Could you check a few things on this model? Use its own coordinates, in mm. A direction names the side the tool comes from. Coordinates: 2 decimals unless noted, no trailing zeros. Loops run counter-clockwise (first coordinate to the right, second up) from the corner with the lowest first, then second, coordinate; pieces in that order, holes last. Notation, with made-up numbers: (86.25, 45.25) - (142.25, 45.25) arc R19 cw to (142.25, 57.25) - close; hole circle Ø9 at (24.25, 14). An arc over 180 degrees is marked (long way). Use CSV: the item, a comma, the result in double quotes.
from build123d import *

# Parameters (mm, degrees)
F1_DEPTH = 2.54
F3_DEPTH = 6.35
F4_W     = 80.137
F4_H     = 207.137
F5_DEPTH = 3.81


with BuildPart() as f1:
    # F0 (on Top) → F1 (new body)
    with BuildSketch(Plane.XY):
        with BuildLine():
            ThreePointArc((0, 1.27), (0.371974, 0.371974), (1.27, 0))
            Line((1.27, 0), (89.535, 0))
            ThreePointArc((89.535, 0), (90.433026, 0.371974), (90.805, 1.27))
            Line((90.805, 1.27), (90.805, 216.535))
            ThreePointArc((90.805, 216.535), (90.433026, 217.433026), (89.535, 217.805))
            Line((89.535, 217.805), (1.27, 217.805))
            ThreePointArc((1.27, 217.805), (0.371974, 217.433026), (0, 216.535))
            Line((0, 216.535), (0, 1.27))
        make_face()
    extrude(amount=F1_DEPTH)

    # F2 (on Top) → F3 (join)
    with BuildSketch(Plane.XY):
        with BuildLine():
            Line((2.794, 213.741), (2.794, 4.064))
            ThreePointArc((2.794, 4.064), (3.165974, 3.165974), (4.064, 2.794))
            Line((4.064, 2.794), (86.741, 2.794))
            ThreePointArc((86.741, 2.794), (87.639026, 3.165974), (88.011, 4.064))
            Line((88.011, 4.064), (88.011, 213.741))
            ThreePointArc((88.011, 213.741), (87.639026, 214.639026), (86.741, 215.011))
            Line((86.741, 215.011), (4.064, 215.011))
            ThreePointArc((4.064, 215.011), (3.165974, 214.639026), (2.794, 213.741))
        make_face()
    extrude(amount=F3_DEPTH)

    # F4 (on face) → F5 (cut)
    with BuildSketch(Plane.XY.offset(6.35)):
        with Locations((45.4025, 108.9025)):
            Rectangle(F4_W, F4_H)
    extrude(amount=-F5_DEPTH, mode=Mode.SUBTRACT)


solid = f1.part
(1) Suppose I cut it at B-B (y = 81). Write out the boundary of the cut face in (x, z) (3 decimals), plus the area to 3 significant figures.
Computed:
outline,"(0, 0) - (90.805, 0) - (90.805, 2.54) - (88.011, 2.54) - (88.011, 6.35) - (85.471, 6.35) - (85.471, 2.54) - (5.334, 2.54) - (5.334, 6.35) - (2.794, 6.35) - (2.794, 2.54) - (0, 2.54) - close"
area,"250 mm²"
(2) Suppose I cut it at A-A (z = 4). Write out the boundary of the cut face in (x, y).
Computed:
outline,"(2.79, 4.06) arc R1.27 ccw to (4.06, 2.79) - (86.74, 2.79) arc R1.27 ccw to (88.01, 4.06) - (88.01, 213.74) arc R1.27 ccw to (86.74, 215.01) - (4.06, 215.01) arc R1.27 ccw to (2.79, 213.74) - close; hole (5.33, 5.33) - (85.47, 5.33) - (85.47, 212.47) - (5.33, 212.47) - close"
(3) Thinking about a two-plate mould opening in Y: for faces 6 (the face through (2.794, 110, 4)), 7 (the face through (45, 2.794, 4)), 8 (the face through (5.334, 107, 4)), which applies, +Y half, -Y half, draft (parallel to the pull), parting line (faces both ways), or undercut?
Computed:
face 6,"draft"
face 7,"-Y half"
face 8,"undercut"
(4) Will these pins go through, and if not, where does the flat tip stop? pin 1 (3 mm diameter, centred on x = 59.5, z = 5, fed in from -Y); pin 2 (24 mm diameter, centred on x = 29.5, y = 78.5, fed in from +Z); pin 3 (1 mm diameter, centred on x = 74.5, z = 5, fed in from +Y).
Computed:
pin 1,"stops at y = 2.79"
pin 2,"stops at z = 2.54"
pin 3,"stops at y = 215.01"
(5) Suppose I cut it at C-C (x = 66). Write out the boundary of the cut face in (y, z) (3 decimals), plus the area to 3 significant figures.
Computed:
outline,"(0, 0) - (217.805, 0) - (217.805, 2.54) - (215.011, 2.54) - (215.011, 6.35) - (212.471, 6.35) - (212.471, 2.54) - (5.334, 2.54) - (5.334, 6.35) - (2.794, 6.35) - (2.794, 2.54) - (0, 2.54) - close"
area,"573 mm²"
(6) Which directions (+Z, -Z, +X, -X, +Y, -Y) give clear straight access to the entire face, cutting with the end or side of a thin tool? Please do faces 1 (the face through (46, 215.011, 4)), 2 (the face through (86, 109, 6.35)), 3 (the face through (45, 110, 0)), 4 (the face through (85.471, 107, 4)), 5 (the face through (88.011, 107, 4)).
Computed:
face 1,"+Z, +X, -X, +Y"
face 2,"+Z, +X, -X, +Y, -Y"
face 3,"-Z, +X, -X, +Y, -Y"
face 4,"+Z"
face 5,"+Z, +X, +Y, -Y"
(7) Please list where these lines run through material, in increasing order: line 1 (Y direction, x = 13, z = 5.75); line 2 (X direction, y = 117, z = 2.75); line 3 (Z direction, x = 35, y = 97).
Computed:
line 1,"y = 2.79 to 5.33, 212.47 to 215.01"
line 2,"x = 2.79 to 5.33, 85.47 to 88.01"
line 3,"z = 0 to 2.54"
